Can you work these out from the drawing? Everything is in mm from the part's minimum corner. Give positions to 0.01 mm unless a question says otherwise; leave off trailing zeros. Loops run counter-clockwise (first coordinate to the right, second up) from the corner with the lowest first, then second, coordinate; pieces in that order, holes last. Notation, with made-up numbers: (45, 72) - (68, 72) arc R14 cw to (68, 85) - close; hole circle Ø1 at (43, 55.5). An arc over 180 degrees is marked (long way). Answer in a Markdown table with one row per item.
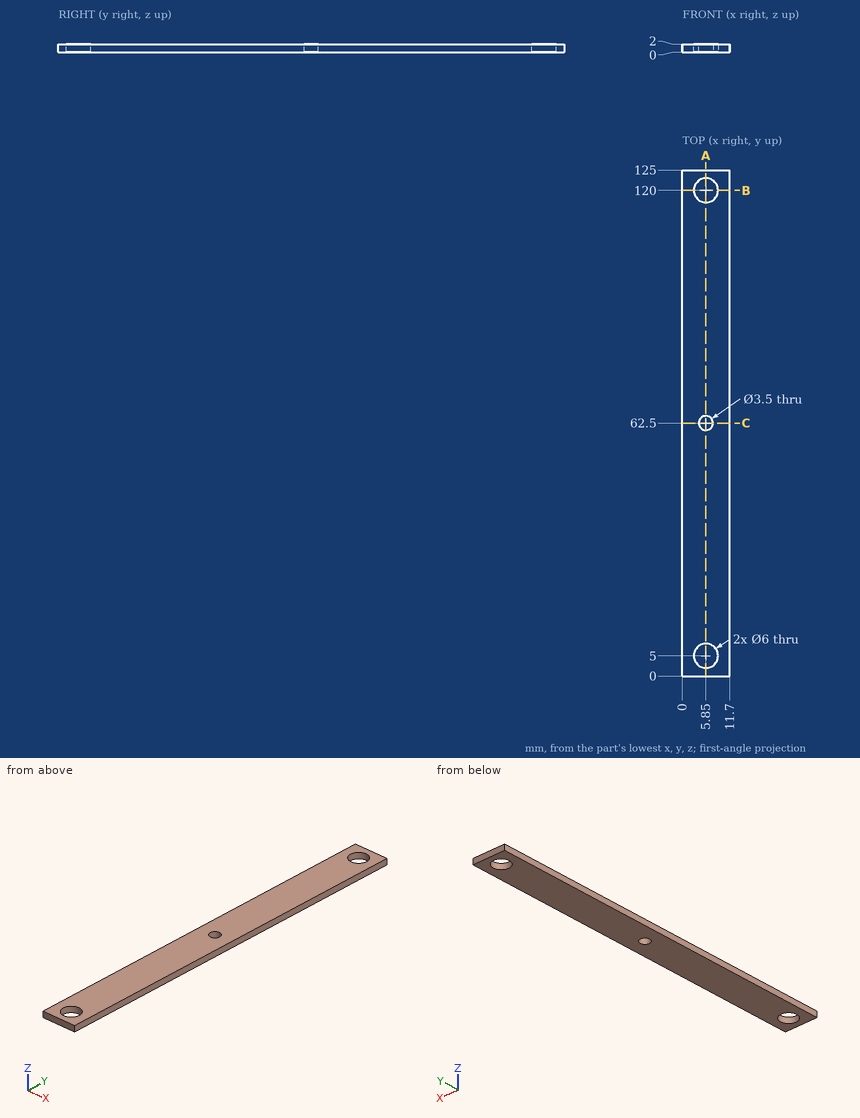
Q1. Imagine slicing it at C-C, the plane y = 62.5. Write out the boundary of the cut face in (x, z).
Checked values:
| item | result |
|---|---|
| outline | (0, 0) - (4.1, 0) - (4.1, 2) - (0, 2) - close; (7.6, 0) - (11.7, 0) - (11.7, 2) - (7.6, 2) - close |
Q2. Imagine slicing it at B-B, the plane y = 120. Write out the boundary of the cut face in (x, z).
Checked values:
| item | result |
|---|---|
| outline | (0, 0) - (2.85, 0) - (2.85, 2) - (0, 2) - close; (8.85, 0) - (11.7, 0) - (11.7, 2) - (8.85, 2) - close |
Q3. If I drill on line 1 (Y direction, x = 5.85, z = 0.5); line 2 (Y direction, x = 6.5, z = 1.1); line 3 (X direction, y = 63.5, z = 1.1), over which ranges is the centre line in solid material (lowest first)? Write a range as [from, to].
Checked values:
| item | result |
|---|---|
| line 1 | y = [0, 2], [8, 60.75], [64.25, 117], [123, 125] |
| line 2 | y = [0, 2.07], [7.93, 60.88], [64.12, 117.07], [122.93, 125] |
| line 3 | x = [0, 4.41], [7.29, 11.7] |
Q4. For pin 1 (3.5 mm diameter, centred on x = 5.85, y = 120, fed in from -Z), with a flat end and sliding along its axis, tell me the tip position at first contact or that it passes through.
Checked values:
| item | result |
|---|---|
| pin 1 | passes through |
Q5. Imagine slicing it at A-A, the plane x = 5.85. Write out the boundary of the cut face in (y, z), and give its area (3 significant figures).
Checked values:
| item | result |
|---|---|
| outline | (0, 0) - (2, 0) - (2, 2) - (0, 2) - close; (8, 0) - (60.75, 0) - (60.75, 2) - (8, 2) - close; (64.25, 0) - (117, 0) - (117, 2) - (64.25, 2) - close; (123, 0) - (125, 0) - (125, 2) - (123, 2) - close |
| area | 219 mm² |
